Study the drawing (mm; zero at the part's minimum x, y, z) and answer. Give positions to 0.01 mm unless a question says otherwise; leave off trailing zeros. Write each loop counter-clockwise with the first axis right and the second up, starting at its lowest first coordinate (ties: lowest second). Pieces come first, ordered by that corner, then holes. Notation, with made-up numbers: M 17,18.5 L 72,18.5 A22 ccw 72,55.5 Z; hole C -1,11 d10. An arc over 180 degrees is marked long. Use a Markdown table: item, result. Add a question column.
Item 1: A cutting plane is placed at D-D on x = 11. Determine the outline of the cut face in (y, z).
Item 2: A cutting plane is placed at C-C on z = 0.7. Determine the outline of the cut face in (x, y), then the cut area to 3 significant figures.
Item 3: Given P1, Ø1.5, axis at x = 11.5, z = 1.5, coming from the -Y side; P2, Ø0.9, axis at y = 9, z = 2, coming from the -X side; P3, Ø1.5, axis at x = 44, z = 2, coming from the +Y side, each flat-ended and moving along its own axis, determine where each tip first touches the part or whether it passes through.
Item 4: A cutting plane is placed at B-B on x = 25.4. Determine the outline of the cut face in (y, z).
Item 5: A cutting plane is placed at A-A on y = 25.5. Determine the outline of the cut face in (x, z).
Item 6: Consider probe 1 along X at (y, z) = (25.5, 1.6); probe 2 along Y at (x, z) = (2, 0.8); probe 3 along Y at (x, z) = (25.4, 0.6). Determine where each line is inside the solid, lowest interval first. Write a range as [from, to].
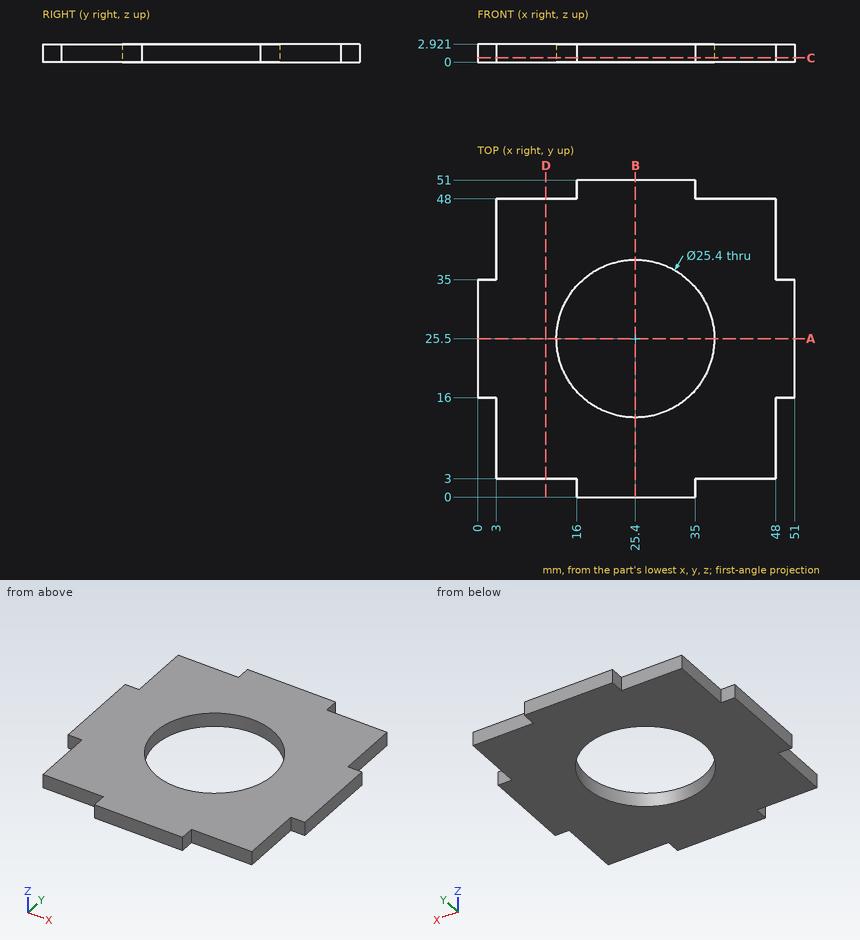
Filled in:
| question | item | result |
|---|---|---|
| 1 | outline | M 3,0 L 48,0 L 48,2.92 L 3,2.92 Z |
| 2 | outline | M 0,16 L 3,16 L 3,3 L 16,3 L 16,0 L 35,0 L 35,3 L 48,3 L 48,16 L 51,16 L 51,35 L 48,35 L 48,48 L 35,48 L 35,51 L 16,51 L 16,48 L 3,48 L 3,35 L 0,35 Z; hole C 25.4,25.5 d25.4 |
| 2 | area | 1,750 mm² |
| 3 | P1 | y = 3 |
| 3 | P2 | x = 3 |
| 3 | P3 | y = 48 |
| 4 | outline | M 0,0 L 12.8,0 L 12.8,2.92 L 0,2.92 Z; M 38.2,0 L 51,0 L 51,2.92 L 38.2,2.92 Z |
| 5 | outline | M 0,0 L 12.7,0 L 12.7,2.92 L 0,2.92 Z; M 38.1,0 L 51,0 L 51,2.92 L 38.1,2.92 Z |
| 6 | probe 1 | [0, 12.7], [38.1, 51] |
| 6 | probe 2 | [16, 35] |
| 6 | probe 3 | [0, 12.8], [38.2, 51] |
